from build123d import *

# Parameters (mm, degrees)
F0_R          = 4.8895
F1_DEPTH      = 19.05
F2_R          = 5.715
F3_DEPTH      = 2.159
F4_R          = 3.4925
F5_DEPTH      = 1.8415
F5_DEPTH_BACK = 1.8415
F6_R          = 8.89
F7_DEPTH      = 25.4
F8_T4_DEPTH   = 13.9953701878
F8_S5_R       = 5.715
F8_T6_DEPTH   = 9
F8_T10_DEPTH  = 13.9953701878
F8_S11_R      = 5.715
F8_T12_DEPTH  = 9
F9_SIZE       = 0.635


# Not quite as in the source:
# - a fillet or chamfer that OpenCascade refuses, or shapes differently, is made with other operations: its cross-section is extruded or revolved along the edge and cut away or added
# - after a boolean that leaves OpenCascade's solid faulty, fix() repairs it


with BuildPart() as f1:
    # F0 (on Top) → F1 (new body)
    with BuildSketch(Plane.XY):
        Circle(F0_R)
    extrude(amount=F1_DEPTH)

    # F2 (on face) → F3 (join)
    with BuildSketch(Plane(origin=(0, 0, 0), x_dir=(1, 0, 0), z_dir=(0, 0, -1))):
        Circle(F2_R)
    extrude(amount=F3_DEPTH)

    # F4 (on Right) → F5 (join, two sides)
    with BuildSketch(Plane.YZ) as f5_sk:
        with BuildLine():
            Line((5.715, -2.159), (-5.715, -2.159))
            Line((-5.715, -2.159), (-5.715, -9.2337771034))
            ThreePointArc((-5.715, -9.2337771034), (0, -13.335), (5.715, -9.2337771034))
            Line((5.715, -9.2337771034), (5.715, -2.159))
        make_face()
        with Locations((0, -7.3025)):
            Circle(F4_R, mode=Mode.SUBTRACT)
    extrude(amount=F5_DEPTH)
    extrude(f5_sk.sketch, amount=-F5_DEPTH_BACK)

    # F6 (on face) → F7 (cut)
    with BuildSketch(Plane(origin=(0, 0, -2.159), x_dir=(1, 0, 0), z_dir=(0, 0, -1))):
        Circle(F6_R)
        with BuildLine():
            ThreePointArc((-1.8415, 5.4101850939), (3.3269394719, 4.6467944596), (5.715, 0))
            ThreePointArc((5.715, 0), (3.3269394719, -4.6467944596), (-1.8415, -5.4101850939))
            ThreePointArc((-1.8415, -5.4101850939), (-5.715, 0), (-1.8415, 5.4101850939))
        make_face(mode=Mode.SUBTRACT)
    extrude(amount=F7_DEPTH, mode=Mode.SUBTRACT)

    add(f1.part.fix(), mode=Mode.REPLACE)

    # F8: fillet of radius 0.635 on 2 edges, made by hand


with BuildPart() as f8_tool2:
    # F8_s3 → F8_t4 (new body)
    with BuildSketch(Plane.XZ.offset(-6.9976850939)):
        with BuildLine():
            ThreePointArc((2.4765, -2.159), (2.0274871939, -2.3449871939), (1.8415, -2.794))
            Line((1.8415, -2.794), (1.8415, -2.159))
            Line((1.8415, -2.159), (2.4765, -2.159))
        make_face()
    extrude(amount=F8_T4_DEPTH)

    # F8_s5 → F8_t6 (intersect, symmetric)
    with BuildSketch(Plane.XY.offset(-2.5)):
        Circle(F8_S5_R)
    extrude(amount=F8_T6_DEPTH, both=True, mode=Mode.INTERSECT)


with BuildPart() as f1_1:
    add(f1.part)

    # F8_t1: union F8_tool2
    add(f8_tool2.part)


with BuildPart() as f8_tool8:
    # F8_s9 → F8_t10 (new body)
    with BuildSketch(Plane.XZ.offset(-6.9976850939)):
        with BuildLine():
            ThreePointArc((-2.4765, -2.159), (-2.0274871939, -2.3449871939), (-1.8415, -2.794))
            Line((-1.8415, -2.794), (-1.8415, -2.159))
            Line((-1.8415, -2.159), (-2.4765, -2.159))
        make_face()
    extrude(amount=F8_T10_DEPTH)

    # F8_s11 → F8_t12 (intersect, symmetric)
    with BuildSketch(Plane.XY.offset(-2.5)):
        Circle(F8_S11_R)
    extrude(amount=F8_T12_DEPTH, both=True, mode=Mode.INTERSECT)


with BuildPart() as f1_2:
    add(f1_1.part)

    # F8_t7: union F8_tool8
    add(f8_tool8.part)

    # F9
    f9_edges = [f1_2.edges().sort_by_distance(p)[0] for p in [
        (-1.8415, -3.4925, -7.3025),
        (1.8415, -3.4925, -7.3025),
    ]]
    chamfer(f9_edges, length=F9_SIZE)


solid = f1_2.part
Could you check a few things on this model? Use its own coordinates, in mm. A direction names the side the tool comes from. Round coordinates to 2 decimals unless told otherwise and drop trailing zeros. Loops run counter-clockwise (first coordinate to the right, second up) from the corner with the lowest first, then second, coordinate; pieces in that order, holes last. Notation, with made-up numbers: (-33, 46) - (14, 46) arc R9 ccw to (14, 54) - close; hole circle Ø9 at (55.5, 84.25). An arc over 180 degrees is marked (long way). Write item = value, one per line.
1) I'm going to push flat-ended pins straight in: P1, Ø5, axis at x = 2, z = 7, coming from the +Y side; P2, Ø3, axis at x = 3.5, z = 12, coming from the +Y side; P3, Ø3, axis at x = -4.5, y = 2.5, coming from the -Z side. Where does each tip first touch, or does it pass through?
Computed:
P1 = 4.89
P2 = 4.46
P3 = -2.16
2) If we mould it in two halves opening along Y, with no side actions, what happens to faces 5 (the flat face through (5, -2, 0)), 6 (the cylindrical face through (-0.02, -0.45, -3.84)), 7 (the cylindrical face through (0.026, -0.105, -13.334))? For each: pulls with the +Y half, pulls with the -Y half, needs draft (parallel to the pull), parting line crosses it, or undercut.
Computed:
face_5 = needs draft
face_6 = undercut
face_7 = parting line crosses it
3) I need wall thicknesses on line 1 along Z through (x, y) = (-0.55, 0) (3 decimals); line 2 along Z through (x, y) = (-5, -1.75); line 3 along Z through (x, y) = (-1.5, 3.25). Which ranges of each line are inside material? Lowest first, please. Write a range as from..to.
Computed:
line_1 = -13.335..-10.795, -3.81..19.05
line_2 = -2.16..0
line_3 = -12.38..-9.24, -5.36..19.05
4) Imagine slicing it at C-C (z = 9.5). Please give me the cut outline in (x, y).
Computed:
outline = circle Ø9.78 at (0, 0)
5) On a 3-axis mill with a long thin cutter (end or side, diameter ignored), from which of +Z, -Z, +X, -X, +Y, -Y can I reach the whole of each face in a straight line? I mean faces 1 (the cylindrical face through (-1.06, -4.773, 9.392)), 2 (the flat face through (1.842, 0, -12)), 3 (the flat face through (-1.842, 0, -12)), 4 (the flat face through (0, 0, 19.05)). Say none if no direction works.
Computed:
face_1 = +Z
face_2 = -Z, +X, +Y, -Y
face_3 = -Z, -X, +Y, -Y
face_4 = +Z, +X, -X, +Y, -Y
